```python
from build123d import *

# Parameters (mm, degrees)
SKETCH1_W                  = 65
SKETCH1_H                  = 65
F_1_4_IN_SHEET_METAL_DEPTH = 3.175
M12_CLEARANCE_HOLE_D       = 12.5
M5_CLEARANCE_HOLE1_D       = 5.3
FILLET1_5_MM_R             = 5
CHAMFER_0_5_MM_SIZE        = 0.5


with BuildPart() as part:
    # Sketch1 → 1/4 in Sheet Metal (new, symmetric)
    with BuildSketch(Plane.XY):
        Rectangle(SKETCH1_W, SKETCH1_H)
    extrude(amount=F_1_4_IN_SHEET_METAL_DEPTH, both=True)

    # M12 Clearance Hole (through all)
    with Locations(Plane.XY.offset(3.175)):
        with Locations((0, 0)):
            Hole(M12_CLEARANCE_HOLE_D / 2)

    # M5 Clearance Hole1 (through all)
    with Locations(Plane.XY.offset(3.175)):
        with Locations((24.748737342, 24.748737342), (-24.748737342, 24.748737342), (-24.748737342, -24.748737342), (24.748737342, -24.748737342)):
            Hole(M5_CLEARANCE_HOLE1_D / 2)

    # Fillet1 5 mm
    fillet1_5_mm_edges = [part.edges().sort_by_distance(p)[0] for p in [
        (32.5, -32.5, 0),
        (-32.5, -32.5, 0),
        (-32.5, 32.5, 0),
        (32.5, 32.5, 0),
    ]]
    fillet(fillet1_5_mm_edges, radius=FILLET1_5_MM_R)

    # Chamfer 0.5 mm
    chamfer_0_5_mm_edges = [part.edges().sort_by_distance(p)[0] for p in [
        (6.25, 0, 3.175),
        (6.25, 0, -3.175),
        (27.398737342, -24.748737342, 3.175),
        (27.398737342, -24.748737342, -3.175),
        (-22.098737342, -24.748737342, 3.175),
        (-22.098737342, -24.748737342, -3.175),
        (-22.098737342, 24.748737342, 3.175),
        (-22.098737342, 24.748737342, -3.175),
        (27.398737342, 24.748737342, 3.175),
        (27.398737342, 24.748737342, -3.175),
    ]]
    chamfer(chamfer_0_5_mm_edges, length=CHAMFER_0_5_MM_SIZE)


solid = part.part
```
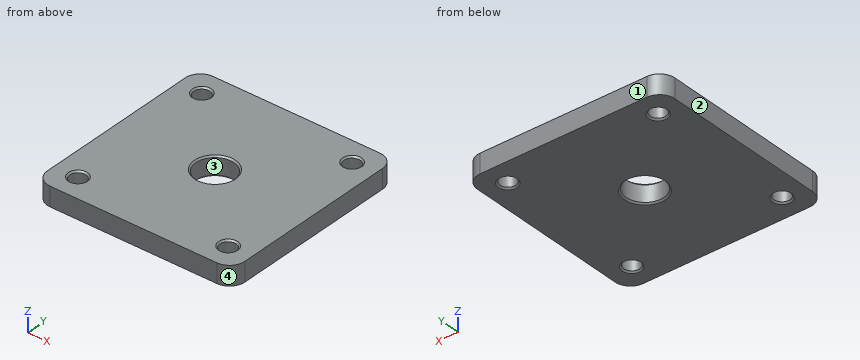
Can you work these out from the model? Positions are in its coordinate system, mm. Face numbers are marked on the shaded views. Give positions to 0.01 mm unless a question says otherwise; leave off trailing zeros. Loops run counter-clockwise (first coordinate to the right, second up) from the corner with the lowest first, then second, coordinate; pieces in that order, holes last. Notation, with made-up numbers: M 29,87.25 L 41,87.25 A7 ccw 41,96.25 Z; hole C 0,60 d3. An arc over 180 degrees is marked long. Use one line per item in the form item = value. Start each with the question number.
(1) I'm going to push flat-ended pins straight in: P1, Ø6, axis at x = -24.75, y = 24.75, coming from the +Z side; P2, Ø10, axis at x = 0, y = 0, coming from the -Z side (1 decimal); P3, Ø6, axis at x = 24.75, y = 24.75, coming from the -Z side. Where does each tip first touch, or does it pass through?
(2) I want a section at D-D, the plane x = -25.5. State how many separate pieces and enclosed holes the cut face has, and give its area (3 significant figures).
(3) I want a section at C-C, the plane z = 1. Write out the boundary of the cut face in (x, y).
(4) Please list where these lines run through material, in increasing order: line 1 (X direction, y = -25, z = 1.25); line 2 (Y direction, x = 0, z = 1.3); line 3 (X direction, y = -23.5, z = 0.75).
(5) Thinking about a two-plate mould opening in Y: for the marked faces 1, 2, 3 and 4, which applies, released by +Y, released by -Y, zero draft, split by the parting line, or undercut?
(6) I want a section at A-A, the plane y = 0. Write out the boundary of the cut face in (x, z) (3 decimals).
Worked out:
q1.P1 = 3.03
q1.P2 = through
q1.P3 = -3.03
q2.separate_pieces = 3
q2.enclosed_holes = 0
q2.area = 347 mm²
q3.outline = M -32.5,-27.5 A5 ccw -27.5,-32.5 L 27.5,-32.5 A5 ccw 32.5,-27.5 L 32.5,27.5 A5 ccw 27.5,32.5 L -27.5,32.5 A5 ccw -32.5,27.5 Z; hole C -24.75,-24.75 d5.3; hole C -24.75,24.75 d5.3; hole C 0,0 d12.5; hole C 24.75,-24.75 d5.3; hole C 24.75,24.75 d5.3
q4.line_1 = -32.5 to -27.39, -22.11 to 22.11, 27.39 to 32.5
q4.line_2 = -32.5 to -6.25, 6.25 to 32.5
q4.line_3 = -32.5 to -27.09, -22.41 to 22.41, 27.09 to 32.5
q5.face_1 = released by +Y
q5.face_2 = zero draft
q5.face_3 = undercut
q5.face_4 = released by -Y
q6.outline = M -32.5,-3.175 L -6.75,-3.175 L -6.25,-2.675 L -6.25,2.675 L -6.75,3.175 L -32.5,3.175 Z; M 6.25,-2.675 L 6.75,-3.175 L 32.5,-3.175 L 32.5,3.175 L 6.75,3.175 L 6.25,2.675 Z
